For this review, use the dimensioned drawing (mm, ordinates from the lowest corner) and the shaded views. A direction names the side the tool comes from. Give positions to 0.01 mm unless a question says otherwise; leave off trailing zeros. Write each loop counter-clockwise with the first axis right and the second up, starting at its lowest first coordinate (ties: lowest second). Pieces come first, ordered by that corner, then holes.
1) Wall thickness on line 1 along Z through (x, y) = (46, 1.5) (3 decimals); line 2 along X through (y, z) = (1, 28); line 3 along X through (y, z) = (3, 30): over which ranges is each line inside the solid? List them lowest first.
2) Machinability: for the marked faces 1 and 2, which of the approach directions +Z, -Z, +X, -X, +Y, -Y give a long, thin tool a straight path to every point of the face, cutting with its end or side? Answer none if there is none.
3) We need section D-D on z = 14.5. Give the boundary of the cut face in (x, y).
4) We need section B-B on y = 4.5. Give the boundary of the cut face in (x, z) (3 decimals), and give its area (3 significant figures).
5) We need section A-A on x = 59. Give the boundary of the cut face in (y, z) (3 decimals), and give its area (3 significant figures).
6) Draft analysis for pull direction X (two halves, no side actions). For the marked faces 3, 4 and 5, state which applies: pulls with the +X half, pulls with the -X half, needs draft (parallel to the pull), parting line crosses it, or undercut.
7) For P1, Ø3, axis at y = 2.5, z = 15.5, coming from the +X side; P2, Ø1.5, axis at y = 1.5, z = 35.5, coming from the -X side; P3, Ø3, axis at x = 11.5, y = 2.5, coming from the +Z side; P4, Ø5.5, axis at x = 74.93, z = 25.4, coming from the +Y side, all flat-tipped, find the tip position at first contact; note any pin that passes through.
8) We need section C-C on z = 25.4. Give the boundary of the cut face in (x, y), and give its area (3 significant figures).
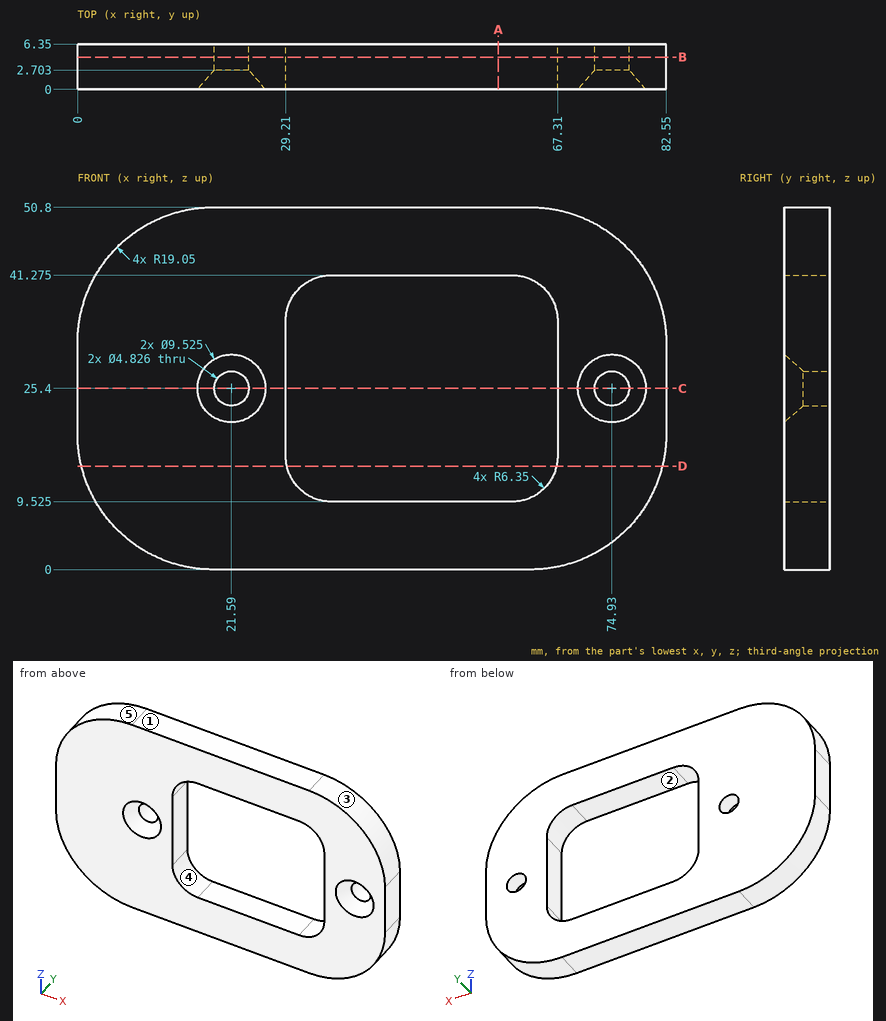
Results list:
1. line 1: z = 0 to 9.525, 41.275 to 50.8
1. line 2: x = 0 to 18.69, 24.49 to 29.21, 67.31 to 72.03, 77.83 to 82.55
1. line 3: x = 0 to 29.21, 67.31 to 82.55
2. face 1: +Z, +X, -X, +Y, -Y
2. face 2: +Y, -Y
3. outline: (0.55, 0) - (29.36, 0) - (29.36, 6.35) - (0.55, 6.35) - close; (67.16, 0) - (82, 0) - (82, 6.35) - (67.16, 6.35) - close
4. outline: (0, 19.05) arc R19.05 ccw to (19.05, 0) - (63.5, 0) arc R19.05 ccw to (82.55, 19.05) - (82.55, 31.75) arc R19.05 ccw to (63.5, 50.8) - (19.05, 50.8) arc R19.05 ccw to (0, 31.75) - close; hole circle Ø4.826 at (21.59, 25.4); hole (29.21, 15.875) arc R6.35 ccw to (35.56, 9.525) - (60.96, 9.525) arc R6.35 ccw to (67.31, 15.875) - (67.31, 34.925) arc R6.35 ccw to (60.96, 41.275) - (35.56, 41.275) arc R6.35 ccw to (29.21, 34.925) - close; hole circle Ø4.826 at (74.93, 25.4)
4. area: 2,670 mm2
5. outline: (0, 0) - (6.35, 0) - (6.35, 9.525) - (0, 9.525) - close; (0, 41.275) - (6.35, 41.275) - (6.35, 50.8) - (0, 50.8) - close
5. area: 121 mm2
6. face 3: pulls with the +X half
6. face 4: undercut
6. face 5: pulls with the -X half
7. P1: stops at x = 82.44
7. P2: stops at x = 0.24
7. P3: stops at z = 49.81
7. P4: stops at y = 6.35
8. outline: (0, 0) - (16.83, 0) - (19.18, 2.7) - (19.18, 6.35) - (0, 6.35) - close; (24, 2.7) - (26.35, 0) - (29.21, 0) - (29.21, 6.35) - (24, 6.35) - close; (67.31, 0) - (70.17, 0) - (72.52, 2.7) - (72.52, 6.35) - (67.31, 6.35) - close; (77.34, 2.7) - (79.69, 0) - (82.55, 0) - (82.55, 6.35) - (77.34, 6.35) - close
8. area: 208 mm2
